Part model, mm, in its own coordinate system. A direction names the side the tool comes from. Coordinates: 2 decimals unless noted, no trailing zeros. Loops run counter-clockwise (first coordinate to the right, second up) from the corner with the lowest first, then second, coordinate; pieces in that order, holes last. Notation, with made-up numbers: M 54.25,-39 L 73.25,-39 A21 ccw 73.25,-4 Z; hole C 77,12 d6. An arc over 180 degrees is marked long. Use a Markdown table: item, result. Add a question column.
1) Tool access for faces 1 (the flat face through (29, 7, -38)), 2 (the flat face through (58, 4, 0)): list every direction of +Z, -Z, +X, -X, +Y, -Y with a clear straight run to the whole face (end or side of a thin tool).
2) Pull direction X, two halves, no side cores. Call faces 3 (the flat face through (-108.5, 4, 0)), 4 (the flat face through (53, 4, -12)), 5 (the flat face through (140, 3, 2)), 6 (the flat face through (29, 0, -38)): released by +X, released by -X, zero draft, split by the parting line, or undercut.
3) Wall check: probe 1 along X at (y, z) = (2.25, -156.5); probe 2 along Z at (x, y) = (-70, 4.25); probe 3 along Z at (x, y) = (-81, 3.25). Give the ranges that are in metal, low to high. Write a range as from..to.
4) Band-saw the part on B-B (y = 3.75). State how many separate pieces and enclosed holes the cut face has, plus the area to 3 significant figures.
5) Band-saw the part on A-A (z = 0). List the corners of the cut face in (x, y).
from build123d import *

# Parameters (mm, degrees)
SKETCH1_W           = 280
SKETCH1_H           = 320
SKETCH1_R           = 1.5
BOSS_EXTRUDE1_DEPTH = 7
SKETCH2_R           = 39
SKETCH2_R_2         = 2.25
SKETCH2_R_3         = 1.5
SKETCH2_W           = 10
SKETCH2_H           = 24
SKETCH2_W_2         = 1.5
SKETCH2_H_2         = 20
CUT_EXTRUDE1_DEPTH  = 10


with BuildPart() as part:
    # Sketch1 → Boss-Extrude1 (new body)
    with BuildSketch(Plane(origin=(0, 0, 0), x_dir=(1, 0, 0), z_dir=(0, 1, 0))):
        Rectangle(SKETCH1_W, SKETCH1_H)
        with Locations(Location((-6.376642336, -156.5, 0), (0, 0, 270))):
            Circle(SKETCH1_R, mode=Mode.SUBTRACT)
        with Locations(Location((-70, 156.5, 0), (0, 0, 270))):
            Circle(SKETCH1_R, mode=Mode.SUBTRACT)
        with Locations(Location((-6.376642336, 156.5, 0), (0, 0, 270))):
            Circle(SKETCH1_R, mode=Mode.SUBTRACT)
        with Locations(Location((70, 156.5, 0), (0, 0, 270))):
            Circle(SKETCH1_R, mode=Mode.SUBTRACT)
        with Locations(Location((70, -156.5, 0), (0, 0, 270))):
            Circle(SKETCH1_R, mode=Mode.SUBTRACT)
        with Locations(Location((-70, -156.5, 0), (0, 0, 270))):
            Circle(SKETCH1_R, mode=Mode.SUBTRACT)
    extrude(amount=BOSS_EXTRUDE1_DEPTH)

    # Sketch2 → Cut-Extrude1 (cut)
    with BuildSketch(Plane(origin=(0, 7, 0), x_dir=(1, 0, 0), z_dir=(0, 1, 0))):
        with Locations(Location((0, 0, 0), (0, 0, 270))):
            Circle(SKETCH2_R)
        with Locations(Location((-35.5, 35.5, 0), (0, 0, 270))):
            Circle(SKETCH2_R_2)
        with Locations(Location((35.5, 35.5, 0), (0, 0, 270))):
            Circle(SKETCH2_R_2)
        with Locations(Location((35.5, -35.5, 0), (0, 0, 270))):
            Circle(SKETCH2_R_2)
        with Locations(Location((-35.5, -35.5, 0), (0, 0, 270))):
            Circle(SKETCH2_R_2)
        with Locations(Location((-107.555652062, 16.833746195, 0), (0, 0, 270))):
            Circle(SKETCH2_R_3)
        with Locations(Location((-81.564347938, 16.833746195, 0), (0, 0, 270))):
            Circle(SKETCH2_R_3)
        with Locations(Location((-107.555652062, -16.833746195, 0), (0, 0, 270))):
            Circle(SKETCH2_R_3)
        with Locations(Location((-81.564347938, -16.833746195, 0), (0, 0, 270))):
            Circle(SKETCH2_R_3)
        with Locations((53, 0)):
            Rectangle(SKETCH2_W, SKETCH2_H)
        with Locations((-109.25, 0)):
            Rectangle(SKETCH2_W_2, SKETCH2_H_2)
    extrude(amount=-CUT_EXTRUDE1_DEPTH, mode=Mode.SUBTRACT)


solid = part.part
Entries:
| question | item | result |
|---|---|---|
| 1 | face 1 | +Z, -Z, +X, -X, +Y |
| 1 | face 2 | +Y, -Y |
| 2 | face 3 | undercut |
| 2 | face 4 | undercut |
| 2 | face 5 | released by +X |
| 2 | face 6 | zero draft |
| 3 | probe 1 | -140..-71.5, -68.5..-7.88, -4.88..68.5, 71.5..140 |
| 3 | probe 2 | -160..-158, -155..155, 158..160 |
| 3 | probe 3 | -160..-18.22, -15.44..15.44, 18.22..160 |
| 4 | separate pieces | 1 |
| 4 | enclosed holes | 17 |
| 4 | area | 84,400 mm2 |
| 5 | outline | M -140,0 L -110,0 L -110,7 L -140,7 Z; M -108.5,0 L -39,0 L -39,7 L -108.5,7 Z; M 39,0 L 48,0 L 48,7 L 39,7 Z; M 58,0 L 140,0 L 140,7 L 58,7 Z |
